Build history of the part. All positions in model axes, mm. Coordinates: 2 decimals unless noted, no trailing zeros. Order: outer loops, then holes, each group sorted by start corner. A loop starts at its lowest first (then second) coordinate and runs counter-clockwise, first axis right, second up. Notation, with made-up numbers: (-8.75, 39) - (27.25, 39) arc R30 ccw to (27.25, 72) - close; hole circle Ø11 at (21.5, 35.25). An arc over 180 degrees is marked (long way). Return JSON: item names as keys, results as strings.
from build123d import *

# Parameters (mm, degrees)
CYLINDER093_R           = 2
CYLINDER093_DEPTH       = 30
CYLINDER019_R           = 1.6
CYLINDER019_DEPTH       = 40
CYLINDER019_PITCH_ANGLE = 90
CYLINDER018_R           = 1.6
CYLINDER018_DEPTH       = 40
CYLINDER018_PITCH_ANGLE = 90
CYLINDER017_R           = 1.6
CYLINDER017_DEPTH       = 40
CYLINDER016_R           = 1.6
CYLINDER016_DEPTH       = 70
CYLINDER016_ROLL_ANGLE  = 90
CYLINDER015_R           = 1.6
CYLINDER015_DEPTH       = 40
BOX013_W                = 116
BOX013_H                = 45
BOX013_DEPTH            = 5


with BuildPart() as cylinder371:
    # Cylinder093 → Cylinder093 (new body)
    with BuildSketch(Plane.XY.offset(128)):
        Circle(CYLINDER093_R)
    extrude(amount=CYLINDER093_DEPTH)


with BuildPart() as cylinder100:
    # Cylinder019 → Cylinder019 (new body)
    with BuildSketch(Plane.XY):
        Circle(CYLINDER019_R)
    extrude(amount=CYLINDER019_DEPTH)


with BuildPart() as cylinder100_1:
    # Cylinder019 pitch: moved
    add(cylinder100.part.rotate(Axis((0, 0, 0), (0, 1, 0)), CYLINDER019_PITCH_ANGLE))


with BuildPart() as cylinder100_2:
    # Cylinder019 placement: moved
    add(cylinder100_1.part.moved(Location((-40, 12, 9.5))))


with BuildPart() as fusion011:
    # Cylinder018 → Cylinder018 (new body)
    with BuildSketch(Plane.XY):
        Circle(CYLINDER018_R)
    extrude(amount=CYLINDER018_DEPTH)


with BuildPart() as fusion011_1:
    # Cylinder018 pitch: moved
    add(fusion011.part.rotate(Axis((0, 0, 0), (0, 1, 0)), CYLINDER018_PITCH_ANGLE))


with BuildPart() as fusion011_2:
    # Cylinder018 placement: moved
    add(fusion011_1.part.moved(Location((-40, -7, 2.5))))

    # Fusion011: union Cylinder100
    add(cylinder100_2.part)


with BuildPart() as fusion012:
    # Cylinder017 → Cylinder017 (new body)
    with BuildSketch(Plane(origin=(-27.5, 7, -15), x_dir=(1, 0, 0), z_dir=(0, 0, 1))):
        Circle(CYLINDER017_R)
    extrude(amount=CYLINDER017_DEPTH)

    # Fusion012: union Fusion011
    add(fusion011_2.part)


with BuildPart() as fusion013:
    # Cylinder016 → Cylinder016 (new body)
    with BuildSketch(Plane.XY):
        Circle(CYLINDER016_R)
    extrude(amount=CYLINDER016_DEPTH)


with BuildPart() as fusion013_1:
    # Cylinder016 roll: moved
    add(fusion013.part.rotate(Axis((0, 0, 0), (1, 0, 0)), CYLINDER016_ROLL_ANGLE))


with BuildPart() as fusion013_2:
    # Cylinder016 placement: moved
    add(fusion013_1.part.moved(Location((-24, 39, 6))))

    # Fusion013: union Fusion012
    add(fusion012.part)


with BuildPart() as cylinder008:
    # Cylinder015 → Cylinder015 (new body)
    with BuildSketch(Plane(origin=(-20.5, -12, -15), x_dir=(1, 0, 0), z_dir=(0, 0, 1))):
        Circle(CYLINDER015_R)
    extrude(amount=CYLINDER015_DEPTH)


with BuildPart() as face_corner_holes014:
    # Fusion028 base: copy of Cylinder008
    add(cylinder008.part)

    # Fusion028: union Fusion013
    add(fusion013_2.part)


with BuildPart() as face_corner_holes014_1:
    # Fusion028 placement: moved
    add(face_corner_holes014.part.moved(Location((104, 0, 132))))


with BuildPart() as face_corner_holes002:
    # Fusion016 base: copy of Cylinder008
    add(cylinder008.part)

    # Fusion016: union Fusion013
    add(fusion013_2.part)


with BuildPart() as face_corner_holes002_1:
    # Fusion016 placement: moved
    add(face_corner_holes002.part.moved(Location((0, 0, 132))))


with BuildPart() as right_a:
    # Box013 → Box013 (new body)
    with BuildSketch(Plane(origin=(-30, -23, 144), x_dir=(1, 0, 0), z_dir=(0, 0, 1))):
        with Locations((58, 22.5)):
            Rectangle(BOX013_W, BOX013_H)
    extrude(amount=BOX013_DEPTH)

    # Cut020: cut face-corner-holes002
    add(face_corner_holes002_1.part, mode=Mode.SUBTRACT)

    # Cut025: cut face-corner-holes014
    add(face_corner_holes014_1.part, mode=Mode.SUBTRACT)

    # Cut053: cut Cylinder371
    add(cylinder371.part, mode=Mode.SUBTRACT)


solid = right_a.part
1. Cut at A-A on x = 76.5. Give the cut face in (y, z).
Check values:
{"outline": "(-23, 144) - (5.4, 144) - (5.4, 149) - (-23, 149) - close; (8.6, 144) - (22, 144) - (22, 149) - (8.6, 149) - close"}
2. Probe L1, parallel to X at y = -12, z = 145.4; L2, parallel to X at y = 7, z = 145.6; L3, parallel to Y at x = 83.5, z = 148.05. List the from-to ranges inside material, lowest first.
Check values:
{"L1": "-30 to -22.1, -18.9 to 81.9, 85.1 to 86", "L2": "-30 to -29.1, -25.9 to 74.9, 78.1 to 86", "L3": "-23 to -13.6, -10.4 to 22"}
3. Cut at B-B on x = 0. Give the cut face in (y, z).
Check values:
{"outline": "(-23, 144) - (-2, 144) - (-2, 149) - (-23, 149) - close; (2, 144) - (22, 144) - (22, 149) - (2, 149) - close"}
4. Drop flat-ended pins along their axis: pin 1 (6.5 mm diameter, centred on x = 0, y = 0, fed in from +Z); pin 2 (1.9 mm diameter, centred on x = -27.5, y = 7, fed in from -Z). Give the stop position or say it passes through.
Check values:
{"pin 1": "z = 149", "pin 2": "through"}
5. Mould opens along Y. For faces 1 (the flat face through (27, -23, 146)), 2 (the cylindrical face through (82.23, -12.97, 146.46)), 3 (the flat face through (86, -1, 146)) say: pulls with the +Y half, pulls with the -Y half, needs draft (parallel to the pull), parting line crosses it, or undercut.
Check values:
{"face 1": "pulls with the -Y half", "face 2": "undercut", "face 3": "needs draft"}
